```python
from build123d import *

# Parameters (mm, degrees)
SKETCH1_R                = 50
SKETCH1_R_2              = 2.5
BOSS_EXTRUDE1_DEPTH      = 5
SKETCH2_R                = 37.5
SKETCH2_R_2              = 33.5
BOSS_EXTRUDE2_DEPTH      = 60
SKETCH3_R                = 33.5
CUT_EXTRUDE1_DEPTH       = 50
BOSS_EXTRUDE4_DEPTH      = 17
BOSS_EXTRUDE4_DEPTH_BACK = 17
SKETCH5_R                = 35
SKETCH5_R_2              = 31
CUT_EXTRUDE2_START       = 10
SKETCH6_R                = 34.5
CUT_EXTRUDE2_DEPTH       = 1.5
CUT_EXTRUDE3_START       = 10
SKETCH7_R                = 35
CUT_EXTRUDE3_DEPTH       = 1.5


with BuildPart() as part:
    # Sketch1 → Boss-Extrude1 (new body)
    with BuildSketch(Plane.XY):
        Circle(SKETCH1_R)
        with Locations((0, 44)):
            Circle(SKETCH1_R_2, mode=Mode.SUBTRACT)
        with Locations((38.105117767, 22)):
            Circle(SKETCH1_R_2, mode=Mode.SUBTRACT)
        with Locations((38.105117767, -22)):
            Circle(SKETCH1_R_2, mode=Mode.SUBTRACT)
        with Locations((0, -44)):
            Circle(SKETCH1_R_2, mode=Mode.SUBTRACT)
        with Locations((-38.105117767, -22)):
            Circle(SKETCH1_R_2, mode=Mode.SUBTRACT)
        with Locations((-38.105117767, 22)):
            Circle(SKETCH1_R_2, mode=Mode.SUBTRACT)
    extrude(amount=BOSS_EXTRUDE1_DEPTH)

    # Sketch2 → Boss-Extrude2 (add)
    with BuildSketch(Plane.XY.offset(5)):
        with Locations(Location((0, 0, 0), (0, 0, 180))):
            Circle(SKETCH2_R)
        with Locations(Location((0, 0, 0), (0, 0, 180))):
            Circle(SKETCH2_R_2, mode=Mode.SUBTRACT)
    extrude(amount=BOSS_EXTRUDE2_DEPTH)

    # Sketch3 → Cut-Extrude1 (cut)
    with BuildSketch(Plane(origin=(0, 0, 0), x_dir=(-1, 0, 0), z_dir=(0, 0, -1))):
        Circle(SKETCH3_R)
    extrude(amount=-CUT_EXTRUDE1_DEPTH, mode=Mode.SUBTRACT)

    # Sketch5 → Boss-Extrude4 (add, two sides: drawn at the far end of the back side and taken through both)
    with BuildSketch(Plane(origin=(0, 0, 32.5), x_dir=(-1, 0, 0), z_dir=(0, 0, -1)).offset(-BOSS_EXTRUDE4_DEPTH_BACK)):
        Circle(SKETCH5_R)
        Circle(SKETCH5_R_2, mode=Mode.SUBTRACT)
    extrude(amount=BOSS_EXTRUDE4_DEPTH + BOSS_EXTRUDE4_DEPTH_BACK)

    # Sketch6 → Cut-Extrude2 (cut)
    with BuildSketch(Plane(origin=(0, 0, 15.5), x_dir=(-1, 0, 0), z_dir=(0, 0, -1)).offset(CUT_EXTRUDE2_START)):
        with Locations(Location((0, 0, 0), (0, 0, 180))):
            Circle(SKETCH6_R)
    extrude(amount=CUT_EXTRUDE2_DEPTH, mode=Mode.SUBTRACT)

    # Sketch7 → Cut-Extrude3 (cut)
    with BuildSketch(Plane.XY.offset(49.5).offset(CUT_EXTRUDE3_START)):
        Circle(SKETCH7_R)
    extrude(amount=CUT_EXTRUDE3_DEPTH, mode=Mode.SUBTRACT)


solid = part.part
```
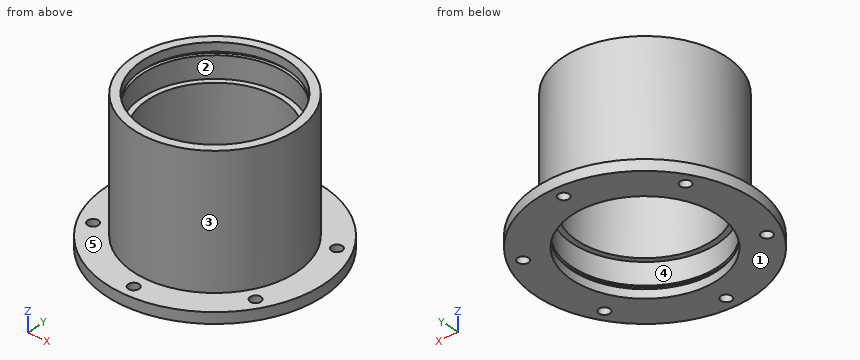
Work out the finished part from the listing and answer in its coordinate system (mm). Face numbers are marked on the shaded views. A direction names the side the tool comes from. Give positions to 0.01 mm unless a question says otherwise; leave off trailing zeros. Order: outer loops, then holes, each group sorted by start corner. A loop starts at its lowest first (then second) coordinate and runs counter-clockwise, first axis right, second up. Notation, with made-up numbers: (55, 19.5) -> (103, 19.5) arc R31 ccw to (103, 54.5) -> close; hole circle Ø2 at (-30.5, 86). An arc over 180 degrees is marked (long way). Answer as CSV lines item,"result". Start each with the question number.
(1) For a pull along Y with two mould halves and no side action, classify the marked faces 3, 4 and 5 as released by +Y, released by -Y, zero draft, split by the parting line, or undercut.
(2) Section B-B, the plane z = 22.5 is taken. Write down the section's boundary in (x, y), plus the area to 3 significant figures.
(3) Each of these flat-tipped pins is pushed along its axis until it touches: pin 1 Ø6 at (y, z) = (5, 39) entering from -X; pin 2 Ø4 at (x, y) = (-38.11, 22) entering from -Z; pin 3 Ø1.5 at (y, z) = (-7.5, 29) entering from -X; pin 4 Ø5 at (x, y) = (37, -26) entering from +Z. Where does it stop, or does it pass through?
(4) Consider line 1 along Y through (x, z) = (-13.5, 41); line 2 along Z through (x, y) = (35.5, -22.5); line 3 along Y through (x, z) = (10.5, 54). Determine where each line is inside the solid, lowest interval first.
(5) Section C-C, the plane y = 44 is taken. Write down the section's boundary in (x, z).
(6) Section A-A, the plane x = 0 is taken. Give the number of separate pieces and of enclosed holes in the cut face, plus the area to 4 significant figures.
(7) Which of the six approach directions +Z, -Z, +X, -X, +Y, -Y give full straight-line access (tool end or side, diameter ignored) to the marked faces 1 and 2?
Entries:
1,face 3,"split by the parting line"
1,face 4,"undercut"
1,face 5,"zero draft"
2,outline,"circle Ø75 at (0, 0); hole circle Ø62 at (0, 0)"
2,area,"1,400 mm²"
3,pin 1,"x = -37.45"
3,pin 2,"through"
3,pin 3,"x = -36.89"
3,pin 4,"z = 5"
4,line 1,"-34.99 to -27.91, 27.91 to 34.99"
4,line 2,"0 to 5"
4,line 3,"-36 to -31.81, 31.81 to 36"
5,outline,"(-23.75, 0) -> (-2.5, 0) -> (-2.5, 5) -> (-23.75, 5) -> close; (2.5, 0) -> (23.75, 0) -> (23.75, 5) -> (2.5, 5) -> close"
6,separate pieces,"4"
6,enclosed holes,"0"
6,area,"757.5 mm²"
7,face 1,"-Z, +X, -X, +Y, -Y"
7,face 2,"+Z"
